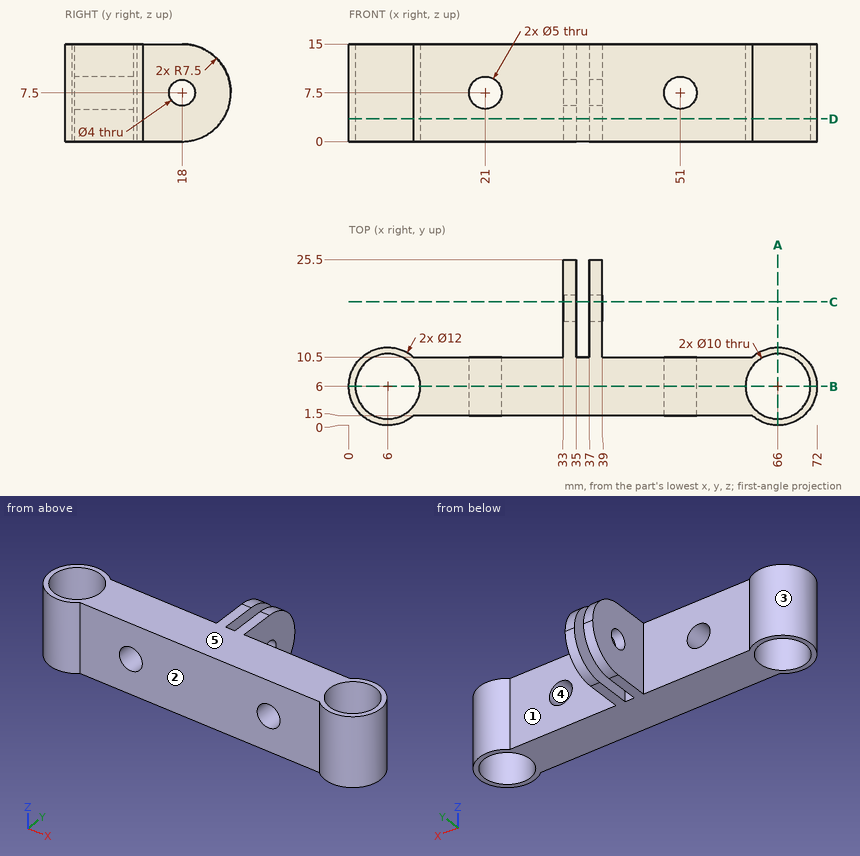
The drawing under review shows one solid part. Ordinate dimensions are in mm from its lowest x, y, z. A direction names the side the tool comes from. Give positions to 0.01 mm unless a question says otherwise; leave off trailing zeros. Write each loop counter-clockwise with the first axis right and the second up, starting at its lowest first coordinate (ties: lowest second). Pieces come first, ordered by that corner, then holes. Notation, with made-up numbers: M -6.5,-13.75 L 17.5,-13.75 A24 cw 17.5,3.25 Z; hole C -21.5,-12 d9. An arc over 180 degrees is marked long. Write each question's results on one line, items separated by ' | '. Start each with the question number.
1. For probe 1 along X at (y, z) = (22, 10); probe 2 along X at (y, z) = (8, 7.5); probe 3 along Y at (x, z) = (66, 4.75), list the stretches that pass through material, from the lowest coordinate up. Write a range as [from, to].
2. We need section C-C (y = 19). Write out the cut boundary in (x, z).
3. We need section D-D (z = 3.5). Write out the cut boundary in (x, y).
4. For the marked faces 1, 2 and 3, list the 3-axis set-ups (+Z, -Z, +X, -X, +Y, -Y) from which the entire face can be reached by the end or side of a thin tool; tool diameter is ignored.
5. Mouldability with a two-part tool opening along X and no side actions: class the marked faces 4 and 5 as released by +X, released by -X, zero draft, split by the parting line, or undercut.
6. We need section B-B (y = 6). Write out the cut boundary in (x, z), and give its area (3 significant figures).
7. We need section A-A (x = 66). Write out the cut boundary in (y, z), and give its area (3 significant figures).
8. Insertion check: pin 1 Ø1 at (y, z) = (15, 10) entering from +X; pin 2 Ø4.5 at (x, z) = (48, 10) entering from +Y; pin 3 Ø5 at (y, z) = (13.5, 4.5) entering from +X. Each pin has a flat end and moves straight along its axis. Give the tip position at first contact, or say it passes through.
Results found:
1) probe 1: x = [33, 35], [37, 39] | probe 2: x = [0.34, 1.42], [10.58, 18.5], [23.5, 48.5], [53.5, 61.42], [70.58, 71.66] | probe 3: y = [0, 1], [11, 12]
2) outline: M 33,0.07 L 35,0.07 L 35,5.77 L 33,5.77 Z; M 33,9.23 L 35,9.23 L 35,14.93 L 33,14.93 Z; M 37,0.07 L 39,0.07 L 39,5.77 L 37,5.77 Z; M 37,9.23 L 39,9.23 L 39,14.93 L 37,14.93 Z
3) outline: M 9.97,1.5 L 62.03,1.5 A6 ccw long 62.03,10.5 L 39,10.5 L 39,24.34 L 37,24.34 L 37,10.5 L 35,10.5 L 35,24.34 L 33,24.34 L 33,10.5 L 9.97,10.5 A6 ccw long Z; hole C 6,6 d10; hole C 66,6 d10
4) face 1: +Z, -Z, +Y | face 2: +Z, -Z, -Y | face 3: +Z, -Z
5) face 4: undercut | face 5: zero draft
6) outline: M 0,0 L 1,0 L 1,15 L 0,15 Z; M 11,0 L 61,0 L 61,15 L 11,15 Z; M 71,0 L 72,0 L 72,15 L 71,15 Z; hole C 21,7.5 d5; hole C 51,7.5 d5 | area: 741 mm^2
7) outline: M 0,0 L 1,0 L 1,15 L 0,15 Z; M 11,0 L 12,0 L 12,15 L 11,15 Z | area: 30.0 mm^2
8) pin 1: stops at x = 39 | pin 2: stops at y = 10.5 | pin 3: stops at x = 69.32
